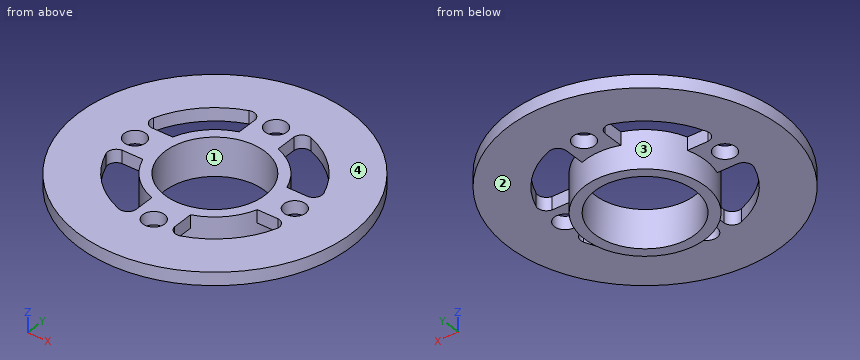
```python
from build123d import *

# Parameters (mm, degrees)
SKETCH2_R                = 52.5
SKETCH2_R_2              = 4.1
BOSS_EXTRUDE1_DEPTH      = 3
SKETCH3_R                = 20.925
CUT_EXTRUDE1_DEPTH       = 9
SKETCH4_R                = 4.5
SKETCH4_R_2              = 2.5
BOSS_EXTRUDE2_DEPTH      = 3
FILLET1_R                = 2
SKETCH5_R                = 52.5
SKETCH5_R_2              = 31.515813439
CUT_EXTRUDE2_DEPTH       = 11.8
BOSS_EXTRUDE3_DEPTH      = 5.8
BOSS_EXTRUDE3_DEPTH_BACK = 3
SKETCH6_R                = 13.925
SKETCH6_R_2              = 11.537787208
BOSS_EXTRUDE4_DEPTH      = 3


with BuildPart() as part:
    # Sketch2 → Boss-Extrude1 (new body)
    with BuildSketch(Plane.XY):
        Circle(SKETCH2_R)
        with Locations((0, 44)):
            Circle(SKETCH2_R_2, mode=Mode.SUBTRACT)
        with Locations((38.105117767, -22)):
            Circle(SKETCH2_R_2, mode=Mode.SUBTRACT)
        with Locations((-38.105117767, -22)):
            Circle(SKETCH2_R_2, mode=Mode.SUBTRACT)
        Polygon((0, 20.207259422), (-17.5, 10.103629711), (-17.5, -10.103629711), (0, -20.207259422), (17.5, -10.103629711), (17.5, 10.103629711), align=None, mode=Mode.SUBTRACT)
    extrude(amount=BOSS_EXTRUDE1_DEPTH)

    # Sketch3 → Cut-Extrude1 (cut)
    with BuildSketch(Plane(origin=(0, 0, 0), x_dir=(-1, 0, 0), z_dir=(0, 0, -1))):
        Circle(SKETCH3_R)
    extrude(amount=-CUT_EXTRUDE1_DEPTH, mode=Mode.SUBTRACT)

    # Sketch4 → Boss-Extrude2 (add)
    # profile 1 of 4: a face of its own
    with BuildSketch(Plane(origin=(0, 0, 0), x_dir=(-1, 0, 0), z_dir=(0, 0, -1))):
        with Locations((0, 18.425)):
            Circle(SKETCH4_R)
        with Locations((0, 18.425)):
            Circle(SKETCH4_R_2, mode=Mode.SUBTRACT)
    # profile 2 of 4: a face of its own
    with BuildSketch(Plane(origin=(0, 0, 0), x_dir=(-1, 0, 0), z_dir=(0, 0, -1))):
        with Locations((-18.425, 0)):
            Circle(SKETCH4_R)
        with Locations((-18.425, 0)):
            Circle(SKETCH4_R_2, mode=Mode.SUBTRACT)
    # profile 3 of 4: a face of its own
    with BuildSketch(Plane(origin=(0, 0, 0), x_dir=(-1, 0, 0), z_dir=(0, 0, -1))):
        with Locations((0, -18.425)):
            Circle(SKETCH4_R)
        with Locations(Location((0, -18.425, 0), (0, 0, 180))):
            Circle(SKETCH4_R_2, mode=Mode.SUBTRACT)
    # profile 4 of 4: a face of its own
    with BuildSketch(Plane(origin=(0, 0, 0), x_dir=(-1, 0, 0), z_dir=(0, 0, -1))):
        with Locations((18.425, 0)):
            Circle(SKETCH4_R)
        with Locations(Location((18.425, 0, 0), (0, 0, 180))):
            Circle(SKETCH4_R_2, mode=Mode.SUBTRACT)
    extrude(amount=-BOSS_EXTRUDE2_DEPTH)

    # Fillet1
    fillet1_edges = [part.edges().sort_by_distance(p)[0] for p in [
        (-3.969288955, 20.545081411, 1.5),
        (3.969288955, 20.545081411, 1.5),
        (20.545081411, 3.969288955, 1.5),
        (20.545081411, -3.969288955, 1.5),
        (3.969288955, -20.545081411, 1.5),
        (-3.969288955, -20.545081411, 1.5),
        (-20.545081411, -3.969288955, 1.5),
        (-20.545081411, 3.969288955, 1.5),
    ]]
    fillet(fillet1_edges, radius=FILLET1_R)

    # Sketch5 → Cut-Extrude2 (cut)
    with BuildSketch(Plane(origin=(0, 0, 0), x_dir=(-1, 0, 0), z_dir=(0, 0, -1))):
        Circle(SKETCH5_R)
        Circle(SKETCH5_R_2, mode=Mode.SUBTRACT)
    extrude(amount=-CUT_EXTRUDE2_DEPTH, mode=Mode.SUBTRACT)



with BuildPart() as body_2:
    # Sketch6 → Boss-Extrude3 (new, two sides: drawn at the far end of the back side and taken through both)
    with BuildSketch(Plane(origin=(0, 0, 0), x_dir=(-1, 0, 0), z_dir=(0, 0, -1)).offset(-BOSS_EXTRUDE3_DEPTH_BACK)):
        Circle(SKETCH6_R)
        Circle(SKETCH6_R_2, mode=Mode.SUBTRACT)
    extrude(amount=BOSS_EXTRUDE3_DEPTH + BOSS_EXTRUDE3_DEPTH_BACK)


with BuildPart() as part_1:
    add(part.part)

    add(body_2.part)  # Boss-Extrude4 merges body 2
    # Sketch7 → Boss-Extrude4 (add)
    with BuildSketch(Plane.XY.offset(3)):
        Polygon((17.982092162, 4.478150583), (13.185286965, 4.478150583), (13.185286965, -4.478150583), (17.982092162, -4.478150583), (17.982092162, -3.600432721), (16.459783373, -2.648989728), (15.103112387, -1.801070362), (15.103112387, 0.78355996), (16.060382876, 2.315192743), (17.5, 3.192690691), align=None)
        Polygon((4.478150583, -17.982092162), (4.478150583, -13.185286965), (-4.478150583, -13.185286965), (-4.478150583, -17.982092162), (-3.600432721, -17.982092162), (-2.648989728, -16.459783373), (-1.801070362, -15.103112387), (0.78355996, -15.103112387), (2.315192743, -16.060382876), (3.192690691, -17.5), align=None)
        Polygon((-17.982092162, -4.478150583), (-13.185286965, -4.478150583), (-13.185286965, 4.478150583), (-17.982092162, 4.478150583), (-17.982092162, 3.600432721), (-16.459783373, 2.648989728), (-15.103112387, 1.801070362), (-15.103112387, -0.78355996), (-16.060382876, -2.315192743), (-17.5, -3.192690691), align=None)
        Polygon((-4.478150583, 17.982092162), (-4.478150583, 13.185286965), (4.478150583, 13.185286965), (4.478150583, 17.982092162), (3.600432721, 17.982092162), (2.648989728, 16.459783373), (1.801070362, 15.103112387), (-0.78355996, 15.103112387), (-2.315192743, 16.060382876), (-3.192690691, 17.5), align=None)
    extrude(amount=-BOSS_EXTRUDE4_DEPTH)


solid = part_1.part
```
Verification items for the finished model (mm, model axes). Face numbers are marked on the shaded views. A direction names the side the tool comes from. Give positions to 0.01 mm unless a question says otherwise; leave off trailing zeros. Order: outer loops, then holes, each group sorted by start corner. A loop starts at its lowest first (then second) coordinate and runs counter-clockwise, first axis right, second up. Notation, with made-up numbers: (20, 70) -> (53, 70) arc R24 cw to (53, 91) -> close; hole circle Ø11 at (-8, 72). An arc over 180 degrees is marked (long way). Use a Markdown table: item, result.
1) Material ranges on probe 1 along Y at (x, z) = (0, -5) (3 decimals); probe 2 along Z at (x, y) = (-26.5, -7.5); probe 3 along Y at (x, z) = (-1.5, -4.75), recorded low to high.
Results:
| item | result |
|---|---|
| probe 1 | -13.925 to -11.538, 11.538 to 13.925 |
| probe 2 | 0 to 3 |
| probe 3 | -13.84 to -11.44, 11.44 to 13.84 |
2) Depth check by flat-ended pin: pin 1 Ø8 at (x, y) = (0, 18.425) entering from -Z; pin 2 Ø3 at (y, z) = (3, -1) entering from -X; pin 3 Ø0.9 at (y, z) = (16.5, 2) entering from -X; pin 4 Ø6.5 at (x, y) = (18.425, 0) entering from +Z. Enter the tip coordinate at first touch or a pass-through.
Results:
| item | result |
|---|---|
| pin 1 | z = 0 |
| pin 2 | x = -31.46 |
| pin 3 | x = -27.12 |
| pin 4 | z = 3 |
3) Mould release check, pull along Y, two halves, no side actions. Record for the marked faces 3 and 4: pulls with the +Y half, pulls with the -Y half, needs draft (parallel to the pull), parting line crosses it, or undercut.
Results:
| item | result |
|---|---|
| face 3 | undercut |
| face 4 | needs draft |
4) Section check D-D, the plane x = -22. Record the boundary of the cut face in (y, z), then the cut area to 3 significant figures.
Results:
| item | result |
|---|---|
| outline | (-22.57, 0) -> (22.57, 0) -> (22.57, 3) -> (-22.57, 3) -> close |
| area | 135 mm² |
5) Tool access check on the marked faces 1 and 2. Record the directions out of +Z, -Z, +X, -X, +Y, -Y that give a thin tool (end or side, any length) a straight path to the whole face; none if there is none.
Results:
| item | result |
|---|---|
| face 1 | +Z, -Z |
| face 2 | -Z |
6) Section check C-C, the plane z = -4.75. Record the boundary of the cut face in (x, y) (3 decimals), then the cut area to 3 significant figures.
Results:
| item | result |
|---|---|
| outline | circle Ø27.85 at (0, 0); hole circle Ø23.076 at (0, 0) |
| area | 191 mm² |
7) Section check A-A, the plane x = 0. Record the boundary of the cut face in (y, z) (3 decimals), then the cut area to 3 significant figures.
Results:
| item | result |
|---|---|
| outline | (-31.516, 0) -> (-20.925, 0) -> (-20.925, 3) -> (-31.516, 3) -> close; (-15.925, 0) -> (-13.925, 0) -> (-13.925, -5.8) -> (-11.538, -5.8) -> (-11.538, 3) -> (-15.925, 3) -> close; (11.538, -5.8) -> (13.925, -5.8) -> (13.925, 0) -> (15.925, 0) -> (15.925, 3) -> (11.538, 3) -> close; (20.925, 0) -> (31.516, 0) -> (31.516, 3) -> (20.925, 3) -> close |
| area | 118 mm² |
